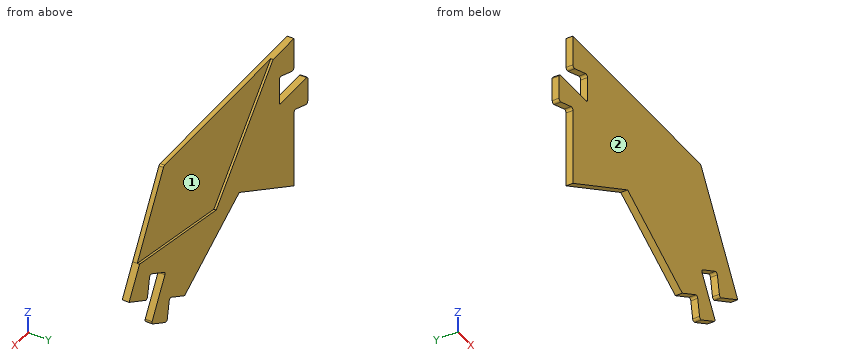
```python
from build123d import *

# Parameters (mm, degrees)
P_IDAT_VYSUNUT_M1_DEPTH = 3
P_IDAT_VYSUNUT_M2_DEPTH = 2
ZAOBLIT1_R              = 1
ZAOBLIT2_R              = 1


with BuildPart() as part:
    # Skica1 → P_idat vysunut_m1 (new body)
    with BuildSketch(Plane(origin=(0, 0, 0), x_dir=(1, 0, 0), z_dir=(0, 1, 0))):
        Polygon((118.524103266, 46.190077074), (105.53372221, 53.690077074), (103.593400635, 42.685966604), (92.248467845, 49.235966604), (102.473720104, 66.946623035), (91.301992395, 73.396623035), (89.463213481, 62.968389614), (78.635106664, 69.22), (39.317553332, 46.52), (0, 69.22), (0, 33.55662508), (-9.950504516, 37.17831254), (-9.950504516, 24.27831254), (10.5, 24.27831254), (10.5, 11.17831254), (0, 15), (0, 0), (15, 0), (55.910618513, 43.889876884), (111.018549767, 33.190077074), align=None)
    extrude(amount=P_IDAT_VYSUNUT_M1_DEPTH)

    # Skica1_3 → P_idat vysunut_m2 (add)
    with BuildSketch(Plane(origin=(0, 0, 0), x_dir=(1, 0, 0), z_dir=(0, 1, 0))):
        Polygon((91.856249834, 0), (111.018549767, 33.190077074), (55.910618513, 43.889876884), (15, 0), align=None)
    extrude(amount=P_IDAT_VYSUNUT_M2_DEPTH)

    # Zaoblit1
    zaoblit1_edges = [part.edges().sort_by_distance(p)[0] for p in [
        (102.473720104, 1.5, -66.946623035),
        (92.248467845, 1.5, -49.235966604),
        (103.593400635, 1.5, -42.685966604),
        (105.53372221, 1.5, -53.690077074),
        (0, 1.5, -15),
        (10.5, 1.5, -11.17831254),
        (10.5, 1.5, -24.27831254),
        (-9.950504516, 1.5, -24.27831254),
        (-9.950504516, 1.5, -37.17831254),
        (0, 1.5, -33.55662508),
        (89.463213481, 1.5, -62.968389614),
        (91.301992395, 1.5, -73.396623035),
    ]]
    fillet(zaoblit1_edges, radius=ZAOBLIT1_R)

    # Zaoblit2
    zaoblit2_edges = [part.edges().sort_by_distance(p)[0] for p in [
        (91.856249834, 1, 0),
    ]]
    fillet(zaoblit2_edges, radius=ZAOBLIT2_R)


solid = part.part
```
The model under review builds one solid part; all positions refer to its coordinate system, in mm. Face numbers are marked on the shaded views. Give positions to 0.01 mm unless a question says otherwise; leave off trailing zeros. Order: outer loops, then holes, each group sorted by start corner. A loop starts at its lowest first (then second) coordinate and runs counter-clockwise, first axis right, second up. Notation, with made-up numbers: (-1, 1.25) - (26, 1.25) arc R6 cw to (26, 5.25) - close; hole circle Ø3 at (-32, 31). An arc over 180 degrees is marked (long way). Use CSV: the item, a comma, the result in double quotes. Start each with the question number.
Q1. We need section D-D, the plane z = -32. Write out the cut boundary in (x, y).
Q2. To check wall thickness, follow line 1 along Y through (x, z) = (31, -17); line 2 along Z through (x, y) = (4, 1.85); line 3 along X through (y, z) = (1.95, -62.5). State the ranges of each line that lie inside material, in increasing order. Write a range as [from, to].
Q3. We need section A-A, the plane z = -57. Write out the cut boundary in (x, y).
Q4. The part is to be moulded in two halves that separate along Y. For the marked faces 1 and 2, say which applies: +Y half, -Y half, draft (parallel to the pull), parting line (faces both ways), or undercut.
Q5. We need section B-B, the plane x = 3. Write out the cut boundary in (y, z), and give its area (3 significant figures).
Q6. Clearance check with flat-ended pins moving along their axes: pin 1 Ø1 at (x, y) = (97, 0.5) entering from -Z; pin 2 Ø0.9 at (y, z) = (1, -53) entering from -X; pin 3 Ø12 at (x, z) = (104.5, -15.5) entering from +Y. State where each tip first meets the part, or that it passes through.
Outcome:
1,outline,"(-9.95, 0) - (110.33, 0) - (110.33, 2) - (44.83, 2) - (44.83, 3) - (-9.95, 3) - close"
2,line 1,"y = [0, 2]"
2,line 2,"z = [-66.91, -24.28], [-13.54, 0]"
2,line 3,"x = [0, 11.64], [67, 99.91]"
3,outline,"(0, 0) - (21.17, 0) - (21.17, 3) - (0, 3) - close; (57.47, 0) - (96.73, 0) - (96.73, 3) - (57.47, 3) - close"
4,face 1,"+Y half"
4,face 2,"-Y half"
5,outline,"(0, -67.49) - (3, -67.49) - (3, -24.28) - (0, -24.28) - close; (0, -13.91) - (3, -13.91) - (3, 0) - (0, 0) - close"
5,area,"171 mm^2"
6,pin 1,"stops at z = -70.4"
6,pin 2,"stops at x = 0"
6,pin 3,"stops at y = 2"
